Design review of the part shown in the three views and the two pictorial views. Dimensions are in mm from the part's minimum x, y and z. A direction names the side the tool comes from. Round coordinates to 2 decimals unless told otherwise and drop trailing zeros. Loops run counter-clockwise (first coordinate to the right, second up) from the corner with the lowest first, then second, coordinate; pieces in that order, holes last.
1. Consider section B-B on y = 52.25. State the section outline as (x, z) points.
2. Consider section A-A on z = 20.25. State the section outline as (x, y) points, then the cut area to 3 significant figures.
3. Tool access review of the marked faces 1 and 2: name each direction out of +Z, -Z, +X, -X, +Y, -Y from which nothing blocks a thin tool from reaching the whole face with its end or side.
4. Consider section C-C on x = 12. State the section outline as (y, z) points, then the cut area to 3 significant figures.
5. Clearance check with flat-ended pins moving along their axes: pin 1 Ø4 at (x, y) = (7, 51.5) entering from +Z; pin 2 Ø1 at (x, y) = (27, 53) entering from +Z. State where each tip first meets the part, or that it passes through.
6. To check wall thickness, follow line 1 along Y through (x, z) = (27.5, 16.25); line 2 along Y through (x, z) = (9, 19.25); line 3 along Z through (x, y) = (52, 53.5). State the ranges of each line that lie inside material, in increasing order.
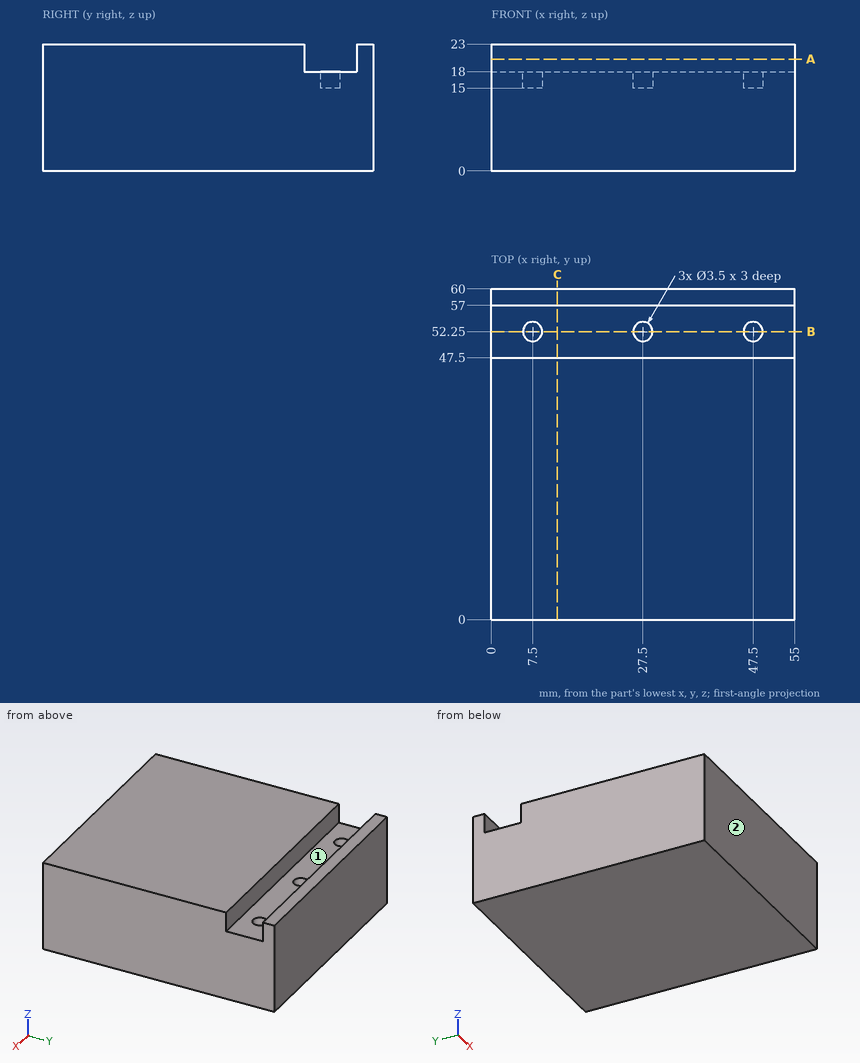
Resolved:
1. outline: (0, 0) - (55, 0) - (55, 18) - (49.25, 18) - (49.25, 15) - (45.75, 15) - (45.75, 18) - (29.25, 18) - (29.25, 15) - (25.75, 15) - (25.75, 18) - (9.25, 18) - (9.25, 15) - (5.75, 15) - (5.75, 18) - (0, 18) - close
2. outline: (0, 0) - (55, 0) - (55, 47.5) - (0, 47.5) - close; (0, 57) - (55, 57) - (55, 60) - (0, 60) - close
2. area: 2,780 mm2
3. face 1: +Z, +X, -X
3. face 2: +Z, -Z, +X, -X, -Y
4. outline: (0, 0) - (60, 0) - (60, 23) - (57, 23) - (57, 18) - (47.5, 18) - (47.5, 23) - (0, 23) - close
4. area: 1,330 mm2
5. pin 1: stops at z = 18
5. pin 2: stops at z = 15
6. line 1: y = 0 to 50.5, 54 to 60
6. line 2: y = 0 to 47.5, 57 to 60
6. line 3: z = 0 to 18
